```python
from build123d import *

# Parameters (mm, degrees)
SKETCH1_R           = 27.5
SKETCH1_R_2         = 22.5
SKETCH1_R_3         = 1.6
BOSS_EXTRUDE1_DEPTH = 11
SKETCH2_R           = 22.5
SKETCH2_R_2         = 21.1
BOSS_EXTRUDE2_DEPTH = 5
SKETCH3_R           = 2
CUT_EXTRUDE1_DEPTH  = 5


with BuildPart() as part:
    # Sketch1 → Boss-Extrude1 (new body)
    with BuildSketch(Plane(origin=(0, 0, 0), x_dir=(1, 0, 0), z_dir=(0, 1, 0))):
        Circle(SKETCH1_R)
        Circle(SKETCH1_R_2, mode=Mode.SUBTRACT)
        with Locations((0, 25)):
            Circle(SKETCH1_R_3, mode=Mode.SUBTRACT)
        with Locations((12.5, 21.650635095)):
            Circle(SKETCH1_R_3, mode=Mode.SUBTRACT)
        with Locations((21.650635095, 12.5)):
            Circle(SKETCH1_R_3, mode=Mode.SUBTRACT)
        with Locations((25, 0)):
            Circle(SKETCH1_R_3, mode=Mode.SUBTRACT)
        with Locations((21.650635095, -12.5)):
            Circle(SKETCH1_R_3, mode=Mode.SUBTRACT)
        with Locations((12.5, -21.650635095)):
            Circle(SKETCH1_R_3, mode=Mode.SUBTRACT)
        with Locations((0, -25)):
            Circle(SKETCH1_R_3, mode=Mode.SUBTRACT)
        with Locations((-12.5, -21.650635095)):
            Circle(SKETCH1_R_3, mode=Mode.SUBTRACT)
        with Locations((-21.650635095, -12.5)):
            Circle(SKETCH1_R_3, mode=Mode.SUBTRACT)
        with Locations((-25, 0)):
            Circle(SKETCH1_R_3, mode=Mode.SUBTRACT)
        with Locations((-21.650635095, 12.5)):
            Circle(SKETCH1_R_3, mode=Mode.SUBTRACT)
        with Locations((-12.5, 21.650635095)):
            Circle(SKETCH1_R_3, mode=Mode.SUBTRACT)
    extrude(amount=BOSS_EXTRUDE1_DEPTH)

    # Sketch2 → Boss-Extrude2 (add)
    with BuildSketch(Plane(origin=(0, 11, 0), x_dir=(1, 0, 0), z_dir=(0, 1, 0))):
        Circle(SKETCH2_R)
        Circle(SKETCH2_R_2, mode=Mode.SUBTRACT)
    extrude(amount=-BOSS_EXTRUDE2_DEPTH)

    # Sketch3 → Cut-Extrude1 (cut)
    with BuildSketch(Plane(origin=(0, 11, 0), x_dir=(1, 0, 0), z_dir=(0, 1, 0))):
        with Locations((0, 25)):
            Circle(SKETCH3_R)
        with Locations((12.5, 21.650635095)):
            Circle(SKETCH3_R)
        with Locations((21.650635095, 12.5)):
            Circle(SKETCH3_R)
        with Locations((25, 0)):
            Circle(SKETCH3_R)
        with Locations((21.650635095, -12.5)):
            Circle(SKETCH3_R)
        with Locations((12.5, -21.650635095)):
            Circle(SKETCH3_R)
        with Locations((0, -25)):
            Circle(SKETCH3_R)
        with Locations((-12.5, -21.650635095)):
            Circle(SKETCH3_R)
        with Locations((-21.650635095, -12.5)):
            Circle(SKETCH3_R)
        with Locations((-25, 0)):
            Circle(SKETCH3_R)
        with Locations((-21.650635095, 12.5)):
            Circle(SKETCH3_R)
        with Locations((-12.5, 21.650635095)):
            Circle(SKETCH3_R)
    extrude(amount=-CUT_EXTRUDE1_DEPTH, mode=Mode.SUBTRACT)


solid = part.part
```
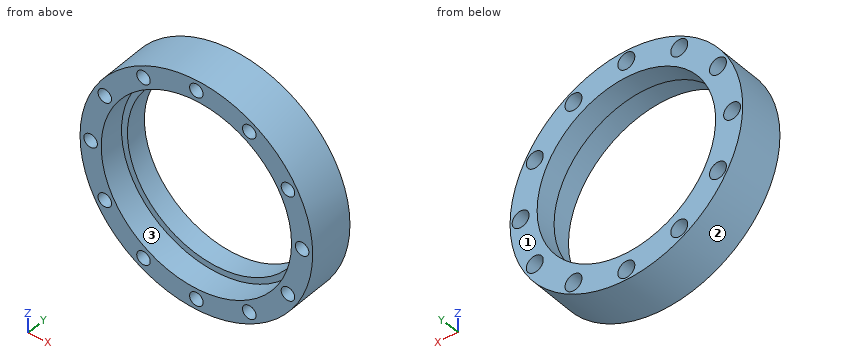
Could you check a few things on this model? Use its own coordinates, in mm. Face numbers are marked on the shaded views. Round coordinates to 2 decimals unless told otherwise and drop trailing zeros. Loops run counter-clockwise (first coordinate to the right, second up) from the corner with the lowest first, then second, coordinate; pieces in that order, holes last.
Q1. I want a section at A-A (x = 0). Write out the boundary of the cut face in (y, z).
Q2. Thinking about a two-plate mould opening in Z: for the marked faces 1, 2 and 3, which applies, pulls with the +Z half, pulls with the -Z half, needs draft (parallel to the pull), parting line crosses it, or undercut?
Q3. I want a section at B-B (z = 0). Write out the boundary of the cut face in (x, y), and give its area (3 significant figures).
Q4. Please list where these lines run through material, in increasing order: L1, parallel to X at y = 7.45, z = 0; L2, parallel to X at y = 3.8, z = 0.
Q5. I want a section at C-C (z = -25). Write out the boundary of the cut face in (x, y).
Q6. I want a section at D-D (x = -25). Write out the boundary of the cut face in (y, z), and give its area (3 significant figures).
Q7. For P1, Ø3, axis at y = 3, z = -4.5, coming from the -X side; P2, Ø4, axis at x = -19.5, y = 8, coming from the +Z side; P3, Ø3, axis at y = 9, z = 17, coming from the -X side, each with a flat end and sliding along its axis, tell me the tip position at first contact or that it passes through.
Answer below:
1. outline: (0, -27.5) - (11, -27.5) - (11, -27) - (6, -27) - (6, -26.6) - (0, -26.6) - close; (0, -23.4) - (6, -23.4) - (6, -23) - (11, -23) - (11, -21.1) - (6, -21.1) - (6, -22.5) - (0, -22.5) - close; (0, 22.5) - (6, 22.5) - (6, 21.1) - (11, 21.1) - (11, 23) - (6, 23) - (6, 23.4) - (0, 23.4) - close; (0, 26.6) - (6, 26.6) - (6, 27) - (11, 27) - (11, 27.5) - (0, 27.5) - close
2. face 1: needs draft
2. face 2: parting line crosses it
2. face 3: undercut
3. outline: (-27.5, 0) - (-26.6, 0) - (-26.6, 6) - (-27, 6) - (-27, 11) - (-27.5, 11) - close; (-23.4, 0) - (-22.5, 0) - (-22.5, 6) - (-21.1, 6) - (-21.1, 11) - (-23, 11) - (-23, 6) - (-23.4, 6) - close; (21.1, 6) - (22.5, 6) - (22.5, 0) - (23.4, 0) - (23.4, 6) - (23, 6) - (23, 11) - (21.1, 11) - close; (26.6, 0) - (27.5, 0) - (27.5, 11) - (27, 11) - (27, 6) - (26.6, 6) - close
3. area: 45.6 mm2
4. L1: x = -27.5 to -27, -23 to -21.1, 21.1 to 23, 27 to 27.5
4. L2: x = -27.5 to -26.6, -23.4 to -22.5, 22.5 to 23.4, 26.6 to 27.5
5. outline: (-11.46, 0) - (-1.6, 0) - (-1.6, 6) - (-2, 6) - (-2, 11) - (-11.46, 11) - close; (1.6, 0) - (11.46, 0) - (11.46, 11) - (2, 11) - (2, 6) - (1.6, 6) - close
6. outline: (0, -11.46) - (11, -11.46) - (11, -2) - (6, -2) - (6, -1.6) - (0, -1.6) - close; (0, 1.6) - (6, 1.6) - (6, 2) - (11, 2) - (11, 11.46) - (0, 11.46) - close
6. area: 213 mm2
7. P1: stops at x = -27.34
7. P2: stops at z = 21.21
7. P3: stops at x = -22.72
